```python
from build123d import *


with BuildPart() as part:
    # Sketch1 → Revolve-Thin1 (revolve)
    with BuildSketch(Plane.XY, mode=Mode.PRIVATE) as revolve_thin1_sk:
        with BuildLine():
            Line((0, 0), (21.427108912, 0))
            ThreePointArc((21.427108912, 0), (22.732446148, 0.484712997), (23.40506946, 1.7039053))
            Line((23.40506946, 1.7039053), (35.5, 82.5))
            Line((35.5, 82.5), (34.708815781, 82.61843788))
            Line((34.708815781, 82.61843788), (22.613885241, 1.82234318))
            ThreePointArc((22.613885241, 1.82234318), (22.210311254, 1.090827798), (21.427108912, 0.8))
            Line((21.427108912, 0.8), (0, 0.8))
            Line((0, 0.8), (0, 0))
        make_face()
    revolve(revolve_thin1_sk.sketch.rotate(Axis((0, 0, 0), (0, 1, 0)), 90), axis=Axis((0, 0, 0), (0, 1, 0)))


solid = part.part
```
Model file for the job. Use its own axes, mm. Coordinates: 2 decimals unless noted, no trailing zeros. Loops run counter-clockwise (first coordinate to the right, second up) from the corner with the lowest first, then second, coordinate; pieces in that order, holes last. Notation, with made-up numbers: (41.25, 85.5) - (84.25, 85.5) arc R22 cw to (84.25, 98.5) - close; hole circle Ø5 at (-13.5, -11.75). An arc over 180 degrees is marked (long way). Answer as a JSON object with one key per item and string values. Group by question number.
(1) Cut at B-B (z = 0). Give the cut face in (x, y), then the cut area to 3 significant figures.
(2) Two-plate mould, pull along Z, no slides. Class faces 1 (the face through (0, 0.8, 0)), 2 (the face through (-1.3, 42.67, 29.51)), 3 (the face through (-28.334, 41.655, 3.72)), 4 (the face through (0, 0, 0)): released by +Z, released by -Z, zero draft, split by the parting line, or undercut.
(3) Cut at A-A (x = 0). Give the cut face in (y, z).
(4) Cut at C-C (y = 72). Give the cut face in (x, z), then the cut area to 3 significant figures.
(5) Flat gauge pins, fed straight in: pin 1 (6 mm diameter, centred on y = 70.5, z = -23, fed in from +X); pin 2 (4 mm diameter, centred on y = 64.5, z = 10.5, fed in from -X); pin 3 (3 mm diameter, centred on x = 28, z = -23.5, fed in from +Y). Where does each tip first touch, or does it go through?
(6) Cut at D-D (y = 39.5). Give the cut face in (x, z), then the cut area to 3 significant figures.
(7) Probe line 1 along Z through (x, y) = (-9.5, 22.5); line 2 along X through (y, z) = (20.5, -1.5); line 3 along X through (y, z) = (11, 7). List the from-to ranges inside material, lowest first.
Geometry says:
{
 "1": {"outline": "(-35.5, 82.5) - (-23.41, 1.7) arc R2 ccw to (-21.43, 0) - (21.43, 0) arc R2 ccw to (23.41, 1.7) - (35.5, 82.5) - (34.71, 82.62) - (22.61, 1.82) arc R1.2 cw to (21.43, 0.8) - (-21.43, 0.8) arc R1.2 cw to (-22.61, 1.82) - (-34.71, 82.62) - close", "area": "169 mm^2"},
 "2": {"face 1": "undercut", "face 2": "split by the parting line", "face 3": "undercut", "face 4": "zero draft"},
 "3": {"outline": "(0, -21.43) arc R2 ccw to (1.7, -23.41) - (82.5, -35.5) - (82.62, -34.71) - (1.82, -22.61) arc R1.2 cw to (0.8, -21.43) - (0.8, 21.43) arc R1.2 cw to (1.82, 22.61) - (82.62, 34.71) - (82.5, 35.5) - (1.7, 23.41) arc R2 ccw to (0, 21.43) - close"},
 "4": {"outline": "circle Ø67.86 at (0, 0); hole circle Ø66.24 at (0, 0)", "area": "170 mm^2"},
 "5": {"pin 1": "stops at x = 27.2", "pin 2": "stops at x = -31.77", "pin 3": "stops at y = 82.57"},
 "6": {"outline": "circle Ø58.13 at (0, 0); hole circle Ø56.51 at (0, 0)", "area": "146 mm^2"},
 "7": {"line 1": "z = -24.76 to -23.89, 23.89 to 24.76", "line 2": "x = -26.18 to -25.37, 25.37 to 26.18", "line 3": "x = -23.79 to -22.94, 22.94 to 23.79"}
}
